Work out the finished part from the listing and answer in its coordinate system (mm). Give positions to 0.01 mm unless a question says otherwise; leave off trailing zeros. Order: outer loops, then holes, each group sorted by start corner. A loop starts at its lowest first (then second) coordinate and runs counter-clockwise, first axis right, second up. Notation, with made-up numbers: (-10.5, -8.75) -> (-5.5, -8.75) arc R9 ccw to (-5.5, -2.75) -> close; hole circle Ø4 at (53, 28). An arc over 180 degrees is marked (long way). Answer as CSV lines item,"result". Start each with the question number.
1. A cutting plane is placed at A-A (x = 59.5). Give the vertices of the cut face in (y, z).
2. Flat-ended cylindrical pins translate along their axes: pin 1 (2.5 mm diameter, centred on x = 628, z = 11, fed in from +Y); pin 2 (12 mm diameter, centred on y = 56, z = 14.5, fed in from -X); pin 3 (5 mm diameter, centred on x = 677, z = 0.5, fed in from +Y). Find the tip coordinate at first contact, or state that the pin passes through.
3. Find the intervals of material crossed by L1, parallel to Y at x = 516.5, z = -6.5; L2, parallel to Y at x = 296, z = -10; L3, parallel to X at y = 100.5, z = 9, in increasing order.
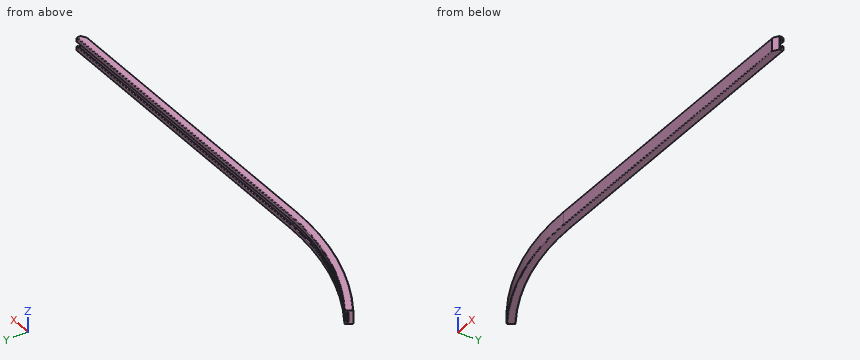
from build123d import *

# Parameters (mm, degrees)
CHAMFER_1_SIZE           = 15
CHAMFER_1_SIZE_2         = 9
CUT_EXTRUDE_1_DEPTH      = 20
CUT_EXTRUDE_1_DEPTH_BACK = 20
SKETCH_3_R               = 3.5
SKETCH_4_R               = 7.5
CUT_EXTRUDE_2_DEPTH      = 10


with BuildPart() as part:
    # По траектории1: sweep along a path in Эскиз1
    with BuildLine(Plane.XY) as sweep_1_path:
        Line((857, 0), (0, 0))
        ThreePointArc((0, 0), (-206.760731281, 29.063109558), (-397.497169801, 114))
    # Эскиз2 → По траектории1 (sweep)
    with BuildSketch(Plane(origin=(857, 0, 0), x_dir=(0, 0, -1), z_dir=(1, 0, 0))):
        with BuildLine():
            Line((11.5, 0), (-11.5, 0))
            ThreePointArc((-11.5, 0), (-12.560660172, 0.439339828), (-13, 1.5))
            Line((-13, 1.5), (-13, 3.5))
            ThreePointArc((-13, 3.5), (-12.560660172, 4.560660172), (-11.5, 5))
            Line((-11.5, 5), (-7, 5))
            ThreePointArc((-7, 5), (-5.939339828, 5.439339828), (-5.5, 6.5))
            Line((-5.5, 6.5), (-5.5, 7.5))
            ThreePointArc((-5.5, 7.5), (-5.939339828, 8.560660172), (-7, 9))
            Line((-7, 9), (-16, 9))
            ThreePointArc((-16, 9), (-17.414213562, 8.414213562), (-18, 7))
            Line((-18, 7), (-18, -9))
            ThreePointArc((-18, -9), (-17.414213562, -10.414213562), (-16, -11))
            Line((-16, -11), (16, -11))
            ThreePointArc((16, -11), (17.414213562, -10.414213562), (18, -9))
            Line((18, -9), (18, 7))
            ThreePointArc((18, 7), (17.414213562, 8.414213562), (16, 9))
            Line((16, 9), (7, 9))
            ThreePointArc((7, 9), (5.939339828, 8.560660172), (5.5, 7.5))
            Line((5.5, 7.5), (5.5, 6.5))
            ThreePointArc((5.5, 6.5), (5.939339828, 5.439339828), (7, 5))
            Line((7, 5), (11.5, 5))
            ThreePointArc((11.5, 5), (12.560660172, 4.560660172), (13, 3.5))
            Line((13, 3.5), (13, 1.5))
            ThreePointArc((13, 1.5), (12.560660172, 0.439339828), (11.5, 0))
        make_face()
    sweep(path=sweep_1_path.line)

    # Фаска1
    # the kernel refuses this chamfer: 15, 9 mm, written as the material it takes off along each edge
    with BuildSketch(Plane(origin=(857, -11, 54.793916458), x_dir=(-0.9998021063601228, -0.019893418958582456, 0), z_dir=(0, 0, -1))) as chamfer_1_piece_1:
        Polygon((CHAMFER_1_SIZE * 0.99980210636, CHAMFER_1_SIZE * 0.0198934189586), (-CHAMFER_1_SIZE_2 * 0.0198934189586, CHAMFER_1_SIZE_2 * 0.99980210636), (0, 0), align=None)
    extrude(amount=109.587832916, mode=Mode.SUBTRACT)

    # Эскиз3 → Вырез-Вытянуть1 (cut, two sides: drawn at the far end of the back side and taken through both)
    with BuildSketch(Plane(origin=(-370.875233434, 98.116911382, 0), x_dir=(0.8691774514901227, -0.4945003112447307, 0), z_dir=(-0.4945003112447307, -0.8691774514901227, 0)).offset(-CUT_EXTRUDE_1_DEPTH_BACK)):
        with Locations(Location((0, 0, 0), (0, 0, 180))):
            Circle(SKETCH_3_R)
    extrude(amount=CUT_EXTRUDE_1_DEPTH + CUT_EXTRUDE_1_DEPTH_BACK, mode=Mode.SUBTRACT)

    # Эскиз4 → Вырез-Вытянуть2 (cut)
    with BuildSketch(Plane(origin=(-50.744094618, -89.192305515, 0), x_dir=(0.8691774514901226, -0.4945003112447307, 0), z_dir=(-0.4945003112447307, -0.8691774514901226, 0))):
        with Locations(Location((-370.875233434, 0, 0), (0, 0, 180))):
            Circle(SKETCH_4_R)
    extrude(amount=CUT_EXTRUDE_2_DEPTH, mode=Mode.SUBTRACT)


solid = part.part
Answer sheet:
1,outline,"(-11, -16) arc R2 ccw to (-9, -18) -> (7, -18) arc R2 ccw to (9, -16) -> (9, -7) arc R1.5 ccw to (7.5, -5.5) -> (6.5, -5.5) arc R1.5 ccw to (5, -7) -> (5, -11.5) arc R1.5 cw to (3.5, -13) -> (1.5, -13) arc R1.5 cw to (0, -11.5) -> (0, 11.5) arc R1.5 cw to (1.5, 13) -> (3.5, 13) arc R1.5 cw to (5, 11.5) -> (5, 7) arc R1.5 ccw to (6.5, 5.5) -> (7.5, 5.5) arc R1.5 ccw to (9, 7) -> (9, 16) arc R2 ccw to (7, 18) -> (-9, 18) arc R2 ccw to (-11, 16) -> close"
2,pin 1,"stops at y = 9"
2,pin 2,"stops at x = -325.23"
2,pin 3,"stops at y = 0"
3,L1,"y = -11 to 0, 5.09 to 8.91"
3,L2,"y = -11 to 0, 5 to 9"
3,L3,"x = -396.57 to -375.03, -364.93 to -356.69"
